from build123d import *

# Parameters (mm, degrees)
F0_W     = 19.05
F0_H     = 19.05
F0_W_2   = 17.018
F0_H_2   = 17.018
F1_DEPTH = 111.252
F2_W     = 3.175
F2_H     = 111.252
F3_DEPTH = 1.016
F4_W     = 18.034
F4_H     = 29.972
F5_DEPTH = 19.051
F6_R     = 0.75057
F7_DEPTH = 19.051


with BuildPart() as f1:
    # F0 (on Top) → F1 (new body)
    with BuildSketch(Plane.XY):
        Rectangle(F0_W, F0_H)
        Rectangle(F0_W_2, F0_H_2, mode=Mode.SUBTRACT)
    extrude(amount=F1_DEPTH)

    # F2 (on face) → F3 (cut, through all)
    with BuildSketch(Plane.XZ.offset(9.525)):
        with Locations((0, 55.626)):
            Rectangle(F2_W, F2_H)
    extrude(amount=-F3_DEPTH, mode=Mode.SUBTRACT)

    # F4 (on face) → F5 (cut, through all)
    with BuildSketch(Plane.YZ.offset(9.525)):
        with Locations((-0.508, 14.986)):
            Rectangle(F4_W, F4_H)
    extrude(amount=-F5_DEPTH, mode=Mode.SUBTRACT)

    # F6 (on face) → F7 (cut, through all)
    with BuildSketch(Plane(origin=(0, 9.525, 0), x_dir=(-1, 0, 0), z_dir=(0, 1, 0))):
        with Locations((0, 12.7)):
            Circle(F6_R)
    extrude(amount=-F7_DEPTH, mode=Mode.SUBTRACT)


solid = f1.part
Source: CAD feature listing. Evaluate the final solid. Frame: model axes, mm. A direction names the side the tool comes from. Round coordinates to 2 decimals unless told otherwise and drop trailing zeros. Loops run counter-clockwise (first coordinate to the right, second up) from the corner with the lowest first, then second, coordinate; pieces in that order, holes last. Notation, with made-up numbers: M 87,12.25 L 143,12.25 A18 cw 143,44.25 Z; hole C -1,-14 d11. An arc over 180 degrees is marked long. Return JSON: item names as keys, results as strings. Group by question number.
1. Section query A-A on y = 1.25. Output: boundary loops of the cut face in (x, z) (3 decimals).
2. Pin query (flat end, axial travel): pin 1 (1.5 mm diameter, centred on x = -7.5, y = -1, fed in from +Z). Return the tip coordinate at first contact, or that it passes through.
3. Reachability of faces 4 (the face through (6, -9.525, 70)), 5 (the face through (9, -3, 29.972)), 6 (the face through (5, -8.509, 70)) from +Z, -Z, +X, -X, +Y, -Y: full face, straight path, thin tool, end or side. Return the list, or none.
4. Mould query, pull axis X, two halves, no side actions, for faces 1 (the face through (8.509, 0, 70)), 2 (the face through (9.525, 0, 67)), 3 (the face through (-9, -4, 29.972)). Classes: released by +X, released by -X, zero draft, split by the parting line, or undercut.
5. Material intervals for line 1 along Y through (x, z) = (5.5, 49) (3 decimals); line 2 along Z through (x, y) = (0, 9), sorted ascending. Write a range as from..to.
6. Section query B-B on x = 7. Output: boundary loops of the cut face in (y, z) (3 decimals), and give its area (3 significant figures).
7. Section query C-C on z = 53. Output: boundary loops of the cut face in (x, y) (1 decimal), and give its area (3 significant figures).
Checks:
{
 "1": {"outline": "M -9.525,29.972 L -8.509,29.972 L -8.509,111.252 L -9.525,111.252 Z; M 8.509,29.972 L 9.525,29.972 L 9.525,111.252 L 8.509,111.252 Z"},
 "2": {"pin 1": "passes through"},
 "3": {"face 4": "+Z, -Z, +X, -X, -Y", "face 5": "-Z, +X, -X, -Y", "face 6": "+Z, -Z"},
 "4": {"face 1": "undercut", "face 2": "released by +X", "face 3": "zero draft"},
 "5": {"line 1": "y = -9.525..-8.509, 8.509..9.525", "line 2": "z = 0..11.95, 13.45..111.25"},
 "6": {"outline": "M -9.525,29.972 L -8.509,29.972 L -8.509,111.252 L -9.525,111.252 Z; M 8.509,0 L 9.525,0 L 9.525,111.252 L 8.509,111.252 Z", "area": "196 mm²"},
 "7": {"outline": "M -9.5,-9.5 L -1.6,-9.5 L -1.6,-8.5 L -8.5,-8.5 L -8.5,8.5 L 8.5,8.5 L 8.5,-8.5 L 1.6,-8.5 L 1.6,-9.5 L 9.5,-9.5 L 9.5,9.5 L -9.5,9.5 Z", "area": "70.1 mm²"}
}
